The model under review builds one solid part; all positions refer to its coordinate system, in mm. A direction names the side the tool comes from. Coordinates: 2 decimals unless noted, no trailing zeros. Order: outer loops, then holes, each group sorted by start corner. A loop starts at its lowest first (then second) coordinate and runs counter-clockwise, first axis right, second up.
```python
from build123d import *

# Parameters (mm, degrees)
SKETCH1_W           = 370
SKETCH1_H           = 150
BOSS_EXTRUDE1_DEPTH = 12
SKETCH3_R           = 37.5
CUT_EXTRUDE2_DEPTH  = 13
SKETCH6_W           = 91
SKETCH6_H           = 8
CUT_EXTRUDE3_DEPTH  = 13
CUT_EXTRUDE4_DEPTH  = 13


with BuildPart() as part:
    # Sketch1 → Boss-Extrude1 (new body)
    with BuildSketch(Plane(origin=(0, 0, 0), x_dir=(1, 0, 0), z_dir=(0, 1, 0))):
        Rectangle(SKETCH1_W, SKETCH1_H)
    extrude(amount=BOSS_EXTRUDE1_DEPTH)

    # Sketch3 → Cut-Extrude2 (cut, through all)
    with BuildSketch(Plane(origin=(0, 12, 0), x_dir=(1, 0, 0), z_dir=(0, 1, 0))):
        Circle(SKETCH3_R)
    extrude(amount=-CUT_EXTRUDE2_DEPTH, mode=Mode.SUBTRACT)

    # Sketch6 → Cut-Extrude3 (cut, through all)
    with BuildSketch(Plane(origin=(0, 12, 0), x_dir=(1, 0, 0), z_dir=(0, 1, 0))):
        Rectangle(SKETCH6_W, SKETCH6_H)
    extrude(amount=-CUT_EXTRUDE3_DEPTH, mode=Mode.SUBTRACT)

    # Sketch7 → Cut-Extrude4 (cut, through all)
    with BuildSketch(Plane(origin=(0, 12, 0), x_dir=(1, 0, 0), z_dir=(0, 1, 0))):
        with BuildLine():
            Line((-150, -58.5), (-172, -58.5))
            ThreePointArc((-172, -58.5), (-176, -62.5), (-172, -66.5))
            Line((-172, -66.5), (-150, -66.5))
            ThreePointArc((-150, -66.5), (-146, -62.5), (-150, -58.5))
        make_face()
        with BuildLine():
            ThreePointArc((-172, 58.5), (-176, 62.5), (-172, 66.5))
            Line((-172, 66.5), (-150, 66.5))
            ThreePointArc((-150, 66.5), (-146, 62.5), (-150, 58.5))
            Line((-150, 58.5), (-172, 58.5))
        make_face()
        with BuildLine():
            ThreePointArc((-117, 58.5), (-121, 62.5), (-117, 66.5))
            Line((-117, 66.5), (-95, 66.5))
            ThreePointArc((-95, 66.5), (-91, 62.5), (-95, 58.5))
            Line((-95, 58.5), (-117, 58.5))
        make_face()
        with BuildLine():
            Line((-95, -58.5), (-117, -58.5))
            ThreePointArc((-117, -58.5), (-121, -62.5), (-117, -66.5))
            Line((-117, -66.5), (-95, -66.5))
            ThreePointArc((-95, -66.5), (-91, -62.5), (-95, -58.5))
        make_face()
    cut_extrude4 = extrude(amount=-CUT_EXTRUDE4_DEPTH, mode=Mode.SUBTRACT)

    # Mirror1: Cut-Extrude4 across plane
    add(cut_extrude4.mirror(Plane(origin=(0, 0, 0), x_dir=(0, 0, 1), z_dir=(1, 0, 0))), mode=Mode.SUBTRACT)


solid = part.part
```
(1) We need section D-D, the plane y = 9.5. Count the separate pieces of the cut face and the enclosed holes in it, and give its area (3 significant figures).
A:
separate pieces: 1
enclosed holes: 9
area: 49,100 mm2
(2) We need section A-A, the plane z = -62.5. Write out the cut boundary in (x, y).
A:
outline: (-185, 0) - (-176, 0) - (-176, 12) - (-185, 12) - close; (-146, 0) - (-121, 0) - (-121, 12) - (-146, 12) - close; (-91, 0) - (91, 0) - (91, 12) - (-91, 12) - close; (121, 0) - (146, 0) - (146, 12) - (121, 12) - close; (176, 0) - (185, 0) - (185, 12) - (176, 12) - close
(3) We need section B-B, the plane x = -161.5. Write out the cut boundary in (y, z), and give its area (3 significant figures).
A:
outline: (0, -75) - (12, -75) - (12, -66.5) - (0, -66.5) - close; (0, -58.5) - (12, -58.5) - (12, 58.5) - (0, 58.5) - close; (0, 66.5) - (12, 66.5) - (12, 75) - (0, 75) - close
area: 1,610 mm2
(4) Draft analysis for pull direction Z (two halves, no side actions). For faces 1 (the face through (41, 6, 4)), 2 (the face through (-146, 6.1, -62.6)), 3 (the face through (185, 6, 1)), 4 (the face through (-3, 6, -75)), state which applies: released by +Z, released by -Z, zero draft, split by the parting line, or undercut.
A:
face 1: undercut
face 2: undercut
face 3: zero draft
face 4: released by -Z
(5) Wall thickness on probe 1 along Z at (x, y) = (-115, 4.5); probe 2 along X at (y, z) = (1.5, 63); probe 3 along X at (y, z) = (8.5, -66): over which ranges is each line inside the solid? List them lowest first.
A:
probe 1: z = -75 to -66.5, -58.5 to 58.5, 66.5 to 75
probe 2: x = -185 to -175.97, -146.03 to -120.97, -91.03 to 91.03, 120.97 to 146.03, 175.97 to 185
probe 3: x = -185 to -173.94, -148.06 to -118.94, -93.06 to 93.06, 118.94 to 148.06, 173.94 to 185
(6) Machinability: for faces 5 (the face through (-3, 6, 75)), 6 (the face through (176, 6.1, -62.4)), which of the approach directions +Z, -Z, +X, -X, +Y, -Y give a long, thin tool a straight path to every point of the face, cutting with its end or side? Answer none if there is none.
A:
face 5: +Z, +X, -X, +Y, -Y
face 6: +Y, -Y
(7) We need section C-C, the plane z = -20. Write out the cut boundary in (x, y).
A:
outline: (-185, 0) - (-31.72, 0) - (-31.72, 12) - (-185, 12) - close; (31.72, 0) - (185, 0) - (185, 12) - (31.72, 12) - close
